```python
from build123d import *

# Parameters (mm, degrees)
SKETCH1_R           = 0.95
BOSS_EXTRUDE1_DEPTH = 4
SKETCH2_W           = 16.2
SKETCH2_H           = 24.45
CUT_EXTRUDE1_DEPTH  = 2


with BuildPart() as part:
    # Sketch1 → Boss-Extrude1 (new body)
    with BuildSketch(Plane.XY):
        with BuildLine():
            Line((0, 17.45), (0, 7))
            Line((0, 7), (4, 7))
            Line((4, 7), (4, 5))
            Line((4, 5), (0, 5))
            Line((0, 5), (0, 2))
            ThreePointArc((0, 2), (0.585786438, 0.585786438), (2, 0))
            Line((2, 0), (14.2, 0))
            ThreePointArc((14.2, 0), (15.614213562, 0.585786438), (16.2, 2))
            Line((16.2, 2), (16.2, 5))
            Line((16.2, 5), (12.2, 5))
            Line((12.2, 5), (12.2, 7))
            Line((12.2, 7), (16.2, 7))
            Line((16.2, 7), (16.2, 17.45))
            Line((16.2, 17.45), (12.2, 17.45))
            Line((12.2, 17.45), (12.2, 19.45))
            Line((12.2, 19.45), (16.2, 19.45))
            Line((16.2, 19.45), (16.2, 22.45))
            ThreePointArc((16.2, 22.45), (15.614213562, 23.864213562), (14.2, 24.45))
            Line((14.2, 24.45), (2, 24.45))
            ThreePointArc((2, 24.45), (0.585786438, 23.864213562), (0, 22.45))
            Line((0, 22.45), (0, 19.45))
            Line((0, 19.45), (4, 19.45))
            Line((4, 19.45), (4, 17.45))
            Line((4, 17.45), (0, 17.45))
        make_face()
        with Locations((13.45, 2.5)):
            Circle(SKETCH1_R, mode=Mode.SUBTRACT)
        with Locations((2.75, 21.95)):
            Circle(SKETCH1_R, mode=Mode.SUBTRACT)
        with Locations((2.75, 2.5)):
            Circle(SKETCH1_R, mode=Mode.SUBTRACT)
        with Locations((13.45, 21.95)):
            Circle(SKETCH1_R, mode=Mode.SUBTRACT)
    extrude(amount=BOSS_EXTRUDE1_DEPTH)

    # Sketch2 → Cut-Extrude1 (cut)
    with BuildSketch(Plane(origin=(0, 0, 0), x_dir=(-1, 0, 0), z_dir=(0, 0, -1))):
        with Locations((-8.1, 12.225)):
            Rectangle(SKETCH2_W, SKETCH2_H)
    extrude(amount=-CUT_EXTRUDE1_DEPTH, mode=Mode.SUBTRACT)


solid = part.part
```
Input: part model. Units: mm. Frame: model coordinates. A direction names the side the tool comes from. Round coordinates to 2 decimals unless told otherwise and drop trailing zeros. Loops run counter-clockwise (first coordinate to the right, second up) from the corner with the lowest first, then second, coordinate; pieces in that order, holes last. Notation, with made-up numbers: (41.25, 22) - (63.25, 22) arc R19 cw to (63.25, 28) - close; hole circle Ø8 at (71.5, 51). An arc over 180 degrees is marked (long way). One line per item, written item: value. Start each with the question number.
(1) Ray query, line 1 (Y direction, x = 13.45, z = 2.6); line 2 (X direction, y = 21.95, z = 3.5); line 3 (X direction, y = 3.25, z = 3.5). Return the intervals inside material, ascending. Write a range as [from, to].
(2) Section B-B, the plane x = 2.75. Return loops of the section in (y, z), plus the area to 3 significant figures.
(3) Contact query for flat-ended pins moving along their axis: P1, Ø0.6, axis at y = 18.5, z = 3.5, coming from the -X side; P2, Ø1, axis at x = 1, z = 3.5, coming from the -Y side; P3, Ø1, axis at y = 18, z = 2.5, coming from the +X side. Output: stop coordinate, or through.
(4) Section D-D, the plane y = 5.75. Return loops of the section in (x, z), plus the area to 3 significant figures.
(5) Section A-A, the plane y = 21.95. Return loops of the section in (x, z), plus the area to 3 significant figures.
(6) Access query for faces 1 (the flat face through (2, 17.45, 3)), 2 (the flat face through (16.2, 21, 3)), 3 (the flat face through (14, 7, 3)). Directions: +Z, -Z, +X, -X, +Y, -Y. A direction counts if a zero-diameter tool reaches every point of the face in a straight line with its end or side. Return the directions, or none.
(7) Section C-C, the plane z = 3.1. Return loops of the section in (x, y).
(8) Draft query along Y for faces 4 (the cylindrical face through (15.63, 23.85, 2.99)), 5 (the flat face through (14, 17.45, 3)), 6 (the cylindrical face through (15.6, 0.57, 2.99)). Return one class per face: +Y half, -Y half, draft (parallel to the pull), parting line (faces both ways), or undercut.
Results below:
1. line 1: [0, 1.55], [3.45, 5], [7, 17.45], [19.45, 21], [22.9, 24.45]
1. line 2: [0, 1.8], [3.7, 12.5], [14.4, 16.2]
1. line 3: [0, 2.17], [3.33, 12.87], [14.03, 16.2]
2. outline: (0, 2) - (1.55, 2) - (1.55, 4) - (0, 4) - close; (3.45, 2) - (5, 2) - (5, 4) - (3.45, 4) - close; (7, 2) - (17.45, 2) - (17.45, 4) - (7, 4) - close; (19.45, 2) - (21, 2) - (21, 4) - (19.45, 4) - close; (22.9, 2) - (24.45, 2) - (24.45, 4) - (22.9, 4) - close
2. area: 33.3 mm^2
3. P1: x = 4
3. P2: y = 0.06
3. P3: x = 12.2
4. outline: (4, 2) - (12.2, 2) - (12.2, 4) - (4, 4) - close
4. area: 16.4 mm^2
5. outline: (0, 2) - (1.8, 2) - (1.8, 4) - (0, 4) - close; (3.7, 2) - (12.5, 2) - (12.5, 4) - (3.7, 4) - close; (14.4, 2) - (16.2, 2) - (16.2, 4) - (14.4, 4) - close
5. area: 24.8 mm^2
6. face 1: +Z, -Z, -X
6. face 2: +Z, -Z, +X, +Y, -Y
6. face 3: +Z, -Z, +X
7. outline: (0, 2) arc R2 ccw to (2, 0) - (14.2, 0) arc R2 ccw to (16.2, 2) - (16.2, 5) - (12.2, 5) - (12.2, 7) - (16.2, 7) - (16.2, 17.45) - (12.2, 17.45) - (12.2, 19.45) - (16.2, 19.45) - (16.2, 22.45) arc R2 ccw to (14.2, 24.45) - (2, 24.45) arc R2 ccw to (0, 22.45) - (0, 19.45) - (4, 19.45) - (4, 17.45) - (0, 17.45) - (0, 7) - (4, 7) - (4, 5) - (0, 5) - close; hole circle Ø1.9 at (2.75, 2.5); hole circle Ø1.9 at (2.75, 21.95); hole circle Ø1.9 at (13.45, 2.5); hole circle Ø1.9 at (13.45, 21.95)
8. face 4: +Y half
8. face 5: undercut
8. face 6: -Y half
